Here's how the part is built. I have some questions about the finished solid (model axes, mm). A direction names the side the tool comes from. Coordinates: 2 decimals unless noted, no trailing zeros. Write each loop counter-clockwise with the first axis right and the second up, starting at its lowest first coordinate (ties: lowest second). Pieces come first, ordered by that corner, then holes. Notation, with made-up numbers: (34.5, 59) -> (75.5, 59) arc R16 cw to (75.5, 73) -> close; hole circle Ø1 at (0, -23.75). An arc over 180 degrees is marked (long way). Use a Markdown table: item, result. Add a question column.
Item 1: Imagine slicing it at D-D, the plane y = -39. Write out the boundary of the cut face in (x, z), and give its area (3 significant figures).
Item 2: Will these pins go through, and if not, where does the flat tip stop? pin 1 Ø1.4 at (x, z) = (13, -3.5) entering from -Y; pin 2 Ø2 at (x, z) = (-13, -4) entering from -Y; pin 3 Ø5 at (y, z) = (-14.5, 1.5) entering from +X.
Item 3: Imagine slicing it at C-C, the plane z = 10.5. Write out the boundary of the cut face in (x, y).
Item 4: Imagine slicing it at B-B, the plane y = -63. Write out the boundary of the cut face in (x, z).
Item 5: If we mould it in two halves opening along X, with no side actions, what happens to faces 3 (the cylindrical face through (-0.069, -66.22, -5.338)), 4 (the flat face through (0, 3.873, -4)), 5 (the flat face through (12, -46.927, -4))? For each: pulls with the +X half, pulls with the -X half, needs draft (parallel to the pull), parting line crosses it, or undercut.
Item 6: Imagine slicing it at A-A, the plane x = 0. Write out the boundary of the cut face in (y, z), and give its area (3 significant figures).
Item 7: If I drill on line 1 along Y through (x, z) = (4, 8); line 2 along Y through (x, z) = (1.5, -4.5); line 3 along X through (y, z) = (-2, -3), over which ranges is the centre line in solid material (lowest first)? Write a range as from..to.
Item 8: On a 3-axis mill with a long thin cutter (end or side, diameter ignored), from which of +Z, -Z, +X, -X, +Y, -Y can I reach the whole of each face in a straight line? I mean faces 1 (the cylindrical face through (17.48, -25.1, -7.66)), 2 (the cylindrical face through (-11.156, -50.146, -4.312)). Say none if no direction works.
```python
from build123d import *

# Parameters (mm, degrees)
F2_R     = 1.397
F3_DEPTH = 6.35


with BuildPart() as f1:
    # F0 (on Right) → F1 (revolve)
    with BuildSketch(Plane.YZ):
        Polygon((-74.35899, -3.777042), (3.87301, -3.777042), (3.87301, 14.129958), (-53.27699, 14.129958), (-53.27699, 2.699958), (-57.84899, 2.699958), (-57.84899, -2.214942), (-74.35899, -2.214942), align=None)
    revolve(axis=Axis((0, -35.24299, -3.777042), (0, -1, 0)))

    # F2 (on face) → F3 (cut)
    with BuildSketch(Plane.XZ.offset(53.27699)):
        with Locations((12.446, -3.777042)):
            Circle(F2_R)
        with Locations((-12.446, -3.777042)):
            Circle(F2_R)
    extrude(amount=-F3_DEPTH, mode=Mode.SUBTRACT)


solid = f1.part
```
Ans:
| question | item | result |
|---|---|---|
| 1 | outline | circle Ø35.81 at (0, -3.78) |
| 1 | area | 1,010 mm^2 |
| 2 | pin 1 | stops at y = -46.93 |
| 2 | pin 2 | stops at y = -53.28 |
| 2 | pin 3 | stops at x = 17.69 |
| 3 | outline | (-10.81, -53.28) -> (10.81, -53.28) -> (10.81, 3.87) -> (-10.81, 3.87) -> close |
| 4 | outline | circle Ø3.12 at (0, -3.78) |
| 5 | face 3 | parting line crosses it |
| 5 | face 4 | needs draft |
| 5 | face 5 | undercut |
| 6 | outline | (-74.36, -5.34) -> (-57.85, -5.34) -> (-57.85, -10.25) -> (-53.28, -10.25) -> (-53.28, -21.68) -> (3.87, -21.68) -> (3.87, 14.13) -> (-53.28, 14.13) -> (-53.28, 2.7) -> (-57.85, 2.7) -> (-57.85, -2.21) -> (-74.36, -2.21) -> close |
| 6 | area | 2,160 mm^2 |
| 7 | line 1 | y = -53.28..3.87 |
| 7 | line 2 | y = -57.85..3.87 |
| 7 | line 3 | x = -17.89..17.89 |
| 8 | face 1 | +Y, -Y |
| 8 | face 2 | -Y |
